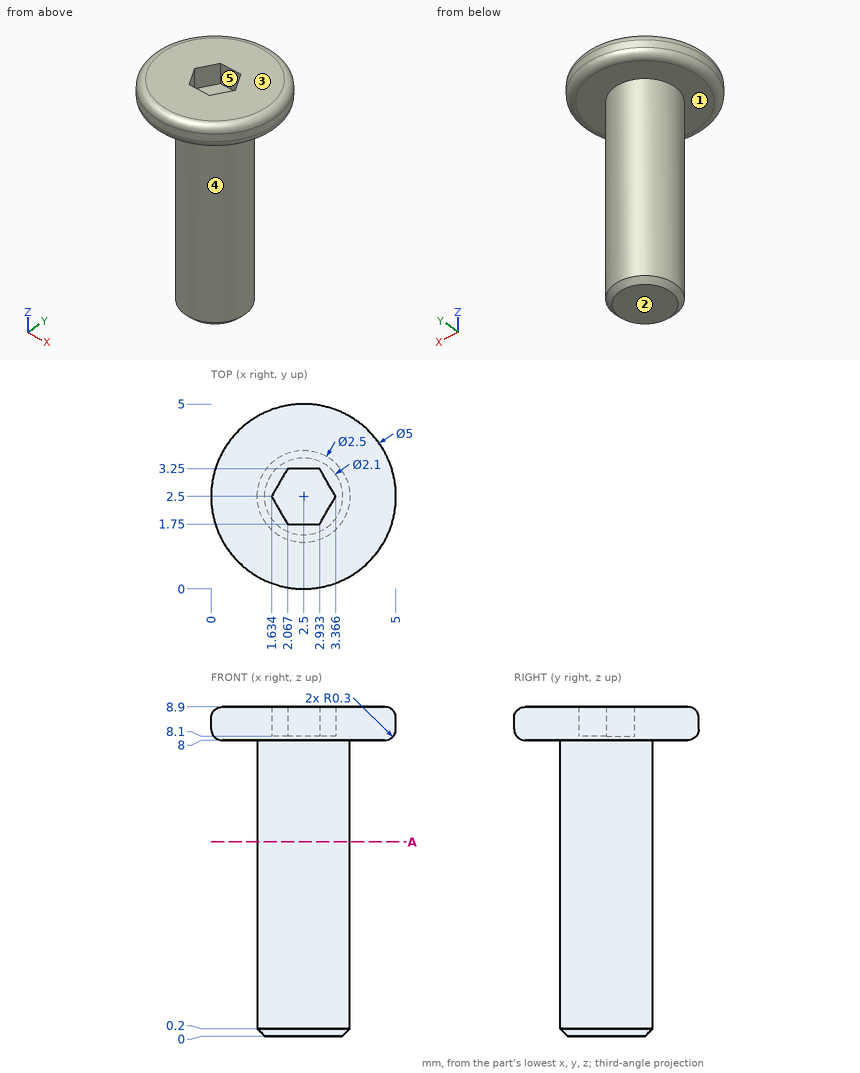
Can you work these out from the drawing? Everything is in mm from the part's minimum corner. A direction names the side the tool comes from. Coordinates: 2 decimals unless noted, no trailing zeros. Loops run counter-clockwise (first coordinate to the right, second up) from the corner with the lowest first, then second, coordinate; pieces in that order, holes last. Notation, with made-up numbers: M -28,8.25 L -19,8.25 A34 cw -19,46.25 Z; hole C 17.25,34 d1. An arc over 180 degrees is marked long. Put each result on its own line as item: value. Start each with the question number.
(1) I need wall thicknesses on line 1 (X direction, y = 3.4, z = 6.5); line 2 (Z direction, x = 3.25, y = 0.9). Which ranges of each line are inside material? Lowest first, please. Write a range as from..to.
(2) Suppose I cut it at A-A on z = 5.25. Please give me the cut outline in (x, y), then the cut area to 3 significant figures.
(3) For the marked faces 1 and 2, which set-ups out of +Z, -Z, +X, -X, +Y, -Y let a thin tool reach every point of the face, with its end or its side?
(4) Thinking about a two-plate mould opening in X: for the marked faces 3, 4 and 5, which applies, pulls with the +X half, pulls with the -X half, needs draft (parallel to the pull), parting line crosses it, or undercut?
Solutions:
1. line 1: x = 1.63..3.37
1. line 2: z = 8..8.9
2. outline: C 2.5,2.5 d2.5
2. area: 4.91 mm2
3. face 1: -Z
3. face 2: -Z, +X, -X, +Y, -Y
4. face 3: needs draft
4. face 4: parting line crosses it
4. face 5: undercut
